CAD build for the part. Positions are in the model's coordinates, mm. A direction names the side the tool comes from. Coordinates: 2 decimals unless noted, no trailing zeros. Loops run counter-clockwise (first coordinate to the right, second up) from the corner with the lowest first, then second, coordinate; pieces in that order, holes last. Notation, with made-up numbers: (-36, -27.75) -> (11, -27.75) arc R7 cw to (11, -17.75) -> close; hole circle Ø10 at (-33.5, 14.5). An arc over 180 degrees is marked (long way). Write item = value, one per line. Start each with the question number.
(1) Pull direction X, two halves, no side cores. Call faces 6 (the face through (-5.323, 12.442, 22.521)), 7 (the face through (-0.232, 30.439, 22.954)), 8 (the face through (13.21, 31.79, 1.97)), 9 (the face through (9.156, 12, 12)): +X half, -X half, draft (parallel to the pull), parting line (faces both ways), or undercut.
(2) Band-saw the part on A-A (z = 16). Write the cut outline in (x, y).
(3) Band-saw the part on D-D (z = 3.5). Write the cut outline in (x, y).
(4) Flat gauge pins, fed straight in: P1, Ø3, axis at x = 16, y = 15.5, coming from the +Z side; P2, Ø8.5, axis at y = 12, z = 10.5, coming from the -X side; P3, Ø1.5, axis at y = -3, z = 5, coming from the +X side. Where does each tip first touch, or does it go through?
(5) Band-saw the part on C-C (x = -1.5). Write the cut outline in (y, z).
(6) Drill centre lines: line 1 (Z direction, x = 1, y = 12.5); line 2 (Y direction, x = 0, z = 22.25); line 3 (Z direction, x = 9.5, y = -7). Where is each one in solid material? Low to high. Write a range as from..to.
(7) Band-saw the part on B-B (y = 9.5). Write the cut outline in (x, z).
(8) Tool access for faces 1 (the face through (14, 13, 4)), 2 (the face through (-16.344, 12, 2)), 3 (the face through (-0.232, 0.439, 22.954)), 4 (the face through (-6.844, 13, 12)), 5 (the face through (-13.02, -6, 1.97)): list every direction of +Z, -Z, +X, -X, +Y, -Y with a clear straight run to the whole face (end or side of a thin tool).
Autodesk Inventor part; units mm, degrees
ref_plane "YZ Plane" through (0, 0, 0) normal (1, 0, 0) x (0, 1, 0)
ref_plane "XZ Plane" through (0, 0, 0) normal (0, 1, 0) x (-1, 0, 0)
ref_plane "XY Plane" through (0, 0, 0) normal (0, 0, 1) x (1, 0, 0)
sketch "Sketch1" plane through (0, 0, 0) normal (0, 0, 1) x (1, 0, 0)
  line L0 (-16.3442, 35.2565) -> (18.6558, 35.2565)
  line L1 (18.6558, 35.2565) -> (18.6558, -9.7435)
  line L2 (18.6558, -9.7435) -> (-16.3442, -9.7435)
  line L3 (-16.3442, -9.7435) -> (-16.3442, 35.2565)
  point P0 (0, 0)
  dimension "d0" = 35
  dimension "d1" = 45
extrude "Extrusion1" add sketch "Sketch1" along normal blind 4
sketch "Sketch2" plane through (0, 0, 4) normal (0, 0, 1) x (1, 0, 0)
  line L0 (-6.8442, -9.7435) -> (9.1558, -9.7435)
  line L1 (9.1558, -9.7435) -> (9.1558, 35.2565)
  line L2 (9.1558, 35.2565) -> (-6.8442, 35.2565)
  line L3 (-6.8442, 35.2565) -> (-6.8442, -9.7435)
  line L4 (-16.3442, -9.7435) -> (18.6558, -9.7435)
  line L5 (18.6558, 35.2565) -> (-16.3442, 35.2565)
  line L6 (-6.8442, 14.4079) -> (-16.3442, 14.4079)
  line L7 (-16.3442, 35.2565) -> (-16.3442, -9.7435)
  line L8 (9.1558, 13.7437) -> (18.6558, 13.7437)
  line L9 (18.6558, -9.7435) -> (18.6558, 35.2565)
  point P0 (0, 0)
  dimension "d4" = 16
extrude "Extrusion2" add sketch "Sketch2" along normal blind 20 contours L3 L2 L1 L0
sketch "Sketch3" plane through (-16.3442, 35.2565, 0) normal (0, 1, 0) x (1, 0, 0)
  circle A0 centre (17.5, -16) radius 6.1
  line L0 (25.5, -4) -> (25.5, -24)
  line L1 (25.5, -24) -> (9.5, -24)
  point P0 (16.3442, 0)
  dimension "d7" = 12.2
  dimension "d8" = 8
  dimension "d9" = 8
extrude "Extrusion3" cut sketch "Sketch3" against normal blind 45
chamfer "Chamfer1" distance 3 angle 45 2 edges at (-6.8442, 12.7565, 24) (9.1558, 12.7565, 24)
sketch "Sketch4" plane through (0, 0, 24) normal (0, 0, 1) x (1, 0, 0)
  line L0 (6.1558, 35.2565) -> (-3.8442, 35.2565)
  line L1 (6.1558, 35.2565) -> (6.1558, -9.7435)
  line L2 (-3.8442, -9.7435) -> (6.1558, -9.7435)
  point P0 (0, 0)
  point P1 (1.1558, 30.2565)
  point P2 (1.1558, 0.2565)
  dimension "d15" = 5
  dimension "d16" = 5
  dimension "d17" = 10
  dimension "d18" = 5
hole "Hole1" at (1.1558, 30.2565, 24) at (1.1558, 0.2565, 24) direction (0, 0, -1) diameter 2.8 depth 10
sketch "Sketch5" plane through (0, 0, 4) normal (0, 0, 1) x (1, 0, 0)
  line L0 (-6.8442, 35.2565) -> (-16.3442, 35.2565)
  line L1 (-16.3442, 35.2565) -> (-16.3442, -9.7435)
  point P0 (0, 0)
  point P1 (-11.8442, 30.7565)
  dimension "d26" = 4.5
  dimension "d27" = 4.5
hole "Hole2" at (-11.8442, 30.7565, 4) direction (0, 0, -1) diameter 2.8 depth 10
pattern_linear "Rectangular Pattern1" count 2 spacing 26 along (1, 0, 0) count 2 spacing 36 along (0, -1, 0) of "Hole2"
properties part number "microscope mount"
Findings below:
q1.face_6 = -X half
q1.face_7 = undercut
q1.face_8 = undercut
q1.face_9 = +X half
q2.outline = (-6.84, -9.74) -> (-4.94, -9.74) -> (-4.94, 35.26) -> (-6.84, 35.26) -> close; (7.26, -9.74) -> (9.16, -9.74) -> (9.16, 35.26) -> (7.26, 35.26) -> close
q3.outline = (-16.34, -9.74) -> (18.66, -9.74) -> (18.66, 35.26) -> (-16.34, 35.26) -> close; hole circle Ø2.8 at (-11.84, -5.24); hole circle Ø2.8 at (-11.84, 30.76); hole circle Ø2.8 at (14.16, -5.24); hole circle Ø2.8 at (14.16, 30.76)
q4.P1 = 4
q4.P2 = -6.84
q4.P3 = 9.16
q5.outline = (-9.74, 0) -> (35.26, 0) -> (35.26, 10.51) -> (-9.74, 10.51) -> close; (-9.74, 21.49) -> (35.26, 21.49) -> (35.26, 24) -> (-9.74, 24) -> close
q6.line_1 = 0..9.9, 22.1..24
q6.line_2 = -9.74..-0.53, 1.05..29.47, 31.05..35.26
q6.line_3 = 0..4
q7.outline = (-16.34, 0) -> (18.66, 0) -> (18.66, 4) -> (9.16, 4) -> (9.16, 21) -> (6.16, 24) -> (-3.84, 24) -> (-6.84, 21) -> (-6.84, 4) -> (-16.34, 4) -> close; hole circle Ø12.2 at (1.16, 16)
q8.face_1 = +Z, +X, +Y, -Y
q8.face_2 = +Z, -Z, -X, +Y, -Y
q8.face_3 = +Z
q8.face_4 = +Z, -X, +Y, -Y
q8.face_5 = +Z, -Z
